from build123d import *

# Parameters (mm, degrees)
SKETCH_1_W               = 44
SKETCH_1_H               = 25
EXTRUDE_1_DEPTH          = 70
SKETCH_2_W               = 22
SKETCH_2_H               = 25
CUT_EXTRUDE_1_DEPTH      = 40
SKETCH_3_R               = 4.5
CUT_EXTRUDE_2_DEPTH      = 50
SKETCH_4_R               = 6.5
CUT_EXTRUDE_4_DEPTH      = 5
SKETCH_5_R               = 3
CUT_EXTRUDE_5_DEPTH      = 29
CUT_EXTRUDE_6_DEPTH      = 5
CUT_EXTRUDE_6_DEPTH_BACK = 5


with BuildPart() as part:
    # Sketch 1 → Extrude 1 (new body)
    with BuildSketch(Plane.XY):
        Rectangle(SKETCH_1_W, SKETCH_1_H)
    extrude(amount=EXTRUDE_1_DEPTH)

    # Sketch 2 → Cut-Extrude 1 (cut)
    with BuildSketch(Plane.XY.offset(70)):
        with Locations((-0.092136373, 0)):
            Rectangle(SKETCH_2_W, SKETCH_2_H)
    extrude(amount=-CUT_EXTRUDE_1_DEPTH, mode=Mode.SUBTRACT)

    # Sketch 3 → Cut-Extrude 2 (cut)
    with BuildSketch(Plane(origin=(22, 0, 0), x_dir=(0, 0, -1), z_dir=(1, 0, 0))):
        with Locations((-52, 3.5)):
            Circle(SKETCH_3_R)
    extrude(amount=-CUT_EXTRUDE_2_DEPTH, mode=Mode.SUBTRACT)

    # Sketch 4 → Cut-Extrude 4 (cut)
    with BuildSketch(Plane.ZY.offset(-22)):
        with Locations((52, 3.5)):
            Circle(SKETCH_4_R)
    cut_extrude_4 = extrude(amount=CUT_EXTRUDE_4_DEPTH, mode=Mode.SUBTRACT)

    # Sketch 5 → Cut-Extrude 5 (cut)
    with BuildSketch(Plane(origin=(0, 12.5, 0), x_dir=(1, 0, 0), z_dir=(0, 1, 0))):
        with Locations(Location((13, -9, 0), (0, 0, 270))):
            Circle(SKETCH_5_R)
        with BuildLine():
            Line((13, 12.355747981), (13, 0))
            ThreePointArc((13, 0), (19.363961031, -2.636038969), (22, -9))
            Line((22, -9), (34.355747981, -9))
            ThreePointArc((34.355747981, -9), (28.100794214, 6.100794214), (13, 12.355747981))
        make_face()
    cut_extrude_5 = extrude(amount=-CUT_EXTRUDE_5_DEPTH, mode=Mode.SUBTRACT)

    # Mirror 2: Cut-Extrude 4, Cut-Extrude 5 across plane
    add(cut_extrude_4.mirror(Plane(origin=(0, 0, 0), x_dir=(0, 0, 1), z_dir=(1, 0, 0))), mode=Mode.SUBTRACT)
    add(cut_extrude_5.mirror(Plane(origin=(0, 0, 0), x_dir=(0, 0, 1), z_dir=(1, 0, 0))), mode=Mode.SUBTRACT)

    # Sketch 6 → Cut-Extrude 6 (cut, two sides: drawn at the far end of the back side and taken through both)
    with BuildSketch(Plane(origin=(0, 0, 0), x_dir=(1, 0, 0), z_dir=(0, 1, 0)).offset(-CUT_EXTRUDE_6_DEPTH_BACK)):
        Polygon((2.5, -19.5), (2.5, 5.258137662), (22, 5.258137662), (22, -14.849242405), (17.349242405, -19.5), align=None)
        Polygon((-22, -14.849242405), (-22, 5.258137662), (-2.5, 5.258137662), (-2.5, -19.5), (-17.349242405, -19.5), align=None)
    extrude(amount=CUT_EXTRUDE_6_DEPTH + CUT_EXTRUDE_6_DEPTH_BACK, mode=Mode.SUBTRACT)


solid = part.part
For this review, take the finished solid that the model builds, in its own axes (mm). A direction names the side the tool comes from. Coordinates: 2 decimals unless noted, no trailing zeros. Loops run counter-clockwise (first coordinate to the right, second up) from the corner with the lowest first, then second, coordinate; pieces in that order, holes last. Notation, with made-up numbers: (-32, 16.5) - (13, 16.5) arc R30 cw to (13, 43.5) - close; hole circle Ø5 at (81.5, 35). An arc over 180 degrees is marked (long way). Return JSON: item names as keys, results as strings.
Item 1: Take a section at D-D (y = 10.75). Give the boundary of the cut face in (x, z).
Determined:
{"outline": "(-22, 9) arc R9 ccw to (-13, 0) - (13, 0) arc R9 ccw to (22, 9) - (22, 70) - (10.91, 70) - (10.91, 30) - (-11.09, 30) - (-11.09, 70) - (-22, 70) - close; hole circle Ø6 at (-13, 9); hole circle Ø6 at (13, 9)"}
Item 2: Take a section at B-B (y = 3.5). State how many separate pieces and enclosed holes the cut face has, then the cut area to 3 significant figures.
Determined:
{"separate pieces": "3", "enclosed holes": "0", "area": "1,220 mm2"}
Item 3: Take a section at A-A (z = 52). Give the boundary of the cut face in (x, y), then the cut area to 3 significant figures.
Determined:
{"outline": "(-22, -12.5) - (-11.09, -12.5) - (-11.09, -1) - (-17, -1) - (-17, -3) - (-22, -3) - close; (-22, 10) - (-17, 10) - (-17, 8) - (-11.09, 8) - (-11.09, 12.5) - (-22, 12.5) - close; (10.91, -12.5) - (22, -12.5) - (22, -3) - (17, -3) - (17, -1) - (10.91, -1) - close; (10.91, 8) - (17, 8) - (17, 10) - (22, 10) - (22, 12.5) - (10.91, 12.5) - close", "area": "312 mm2"}
Item 4: For faces 4 (the flat face through (-2.5, 0, 10)), 5 (the flat face through (0, 0, 30)), 6 (the flat face through (17, -1, 50)), list the 3-axis set-ups (+Z, -Z, +X, -X, +Y, -Y) from which the entire face can be reached by the end or side of a thin tool; tool diameter is ignored.
Determined:
{"face 4": "-Z", "face 5": "+Z, +Y, -Y", "face 6": "+X"}
Item 5: Take a section at C-C (x = 6.5). Give the boundary of the cut face in (y, z).
Determined:
{"outline": "(-12.5, 0) - (-5, 0) - (-5, 19.5) - (5, 19.5) - (5, 0) - (12.5, 0) - (12.5, 30) - (-12.5, 30) - close"}
Item 6: For line 1 (X direction, y = -6.75, z = 9); line 2 (Z direction, x = -13, y = 7.5); line 3 (X direction, y = 11, z = 50), list the stretches that pass through material, from the lowest coordinate up.
Determined:
{"line 1": "x = -22 to -16, -10 to 10, 16 to 22", "line 2": "z = 0 to 6, 12 to 49.94, 54.06 to 70", "line 3": "x = -22 to -11.09, 10.91 to 22"}
Item 7: Mouldability with a two-part tool opening along Y and no side actions: class faces 1 (the flat face through (16, 0, 70)), 2 (the flat face through (10, 5, 12)), 3 (the flat face through (0, -12.5, 27)) as pulls with the +Y half, pulls with the -Y half, needs draft (parallel to the pull), parting line crosses it, or undercut.
Determined:
{"face 1": "needs draft", "face 2": "undercut", "face 3": "pulls with the -Y half"}
Item 8: Insertion check: pin 1 (4 mm diameter, centred on y = 6, z = 49, fed in from +X); pin 2 (3 mm diameter, centred on x = 7, y = 2.5, fed in from -Z). Each pin has a flat end and moves straight along its axis. Give the tip position at first contact, or say it passes through.
Determined:
{"pin 1": "stops at x = 17", "pin 2": "stops at z = 19.5"}
